from build123d import *

# Parameters (mm, degrees)
SKETCH2_W                      = 230
SKETCH2_H                      = 283.251
BOSS_EXTRUDE1_DEPTH            = 10
SKETCH3_W                      = 10
SKETCH3_H                      = 283.251
BOSS_EXTRUDE2_DEPTH            = 170
M6_CLEARANCE_HOLE1_D           = 7
CUT_EXTRUDE1_DEPTH             = 327.431895271
CUT_EXTRUDE1_DEPTH_BACK        = 327.431895271
SKETCH7_R                      = 3.81
SKETCH7_R_2                    = 1.89865
SKETCH8_W                      = 6.35
SKETCH8_H                      = 38.1
CUT_EXTRUDE2_DEPTH             = 36.025
CUT_EXTRUDE3_DEPTH             = 6.35
CUT_EXTRUDE4_REACH             = 331.125
SKETCH11_R                     = 3.81
F_6_CLEARANCE_HOLE1_D          = 3.7973
F_6_CLEARANCE_HOLE1_DEPTH      = 3.65
CIRPATTERN1_COUNT              = 2
ENL_V_MAT_EXTRU_1_REACH        = 249.554
ESQUISSE1_R                    = 3.175
CBORE_FOR_M5_SHCS1_D           = 5.5
CBORE_FOR_M5_SHCS1_CBORE_D     = 10
CBORE_FOR_M5_SHCS1_CBORE_DEPTH = 5
CUT_EXTRUDE5_DEPTH             = 248.553594703
CUT_EXTRUDE5_DEPTH_BACK        = 248.553594703
SKETCH15_W                     = 58.825
SKETCH15_H                     = 30.860637148
CUT_EXTRUDE7_DEPTH             = 248.553594703
CUT_EXTRUDE7_DEPTH_BACK        = 248.553594703
SKETCH20_W                     = 0.765
SKETCH20_H                     = 30.860637148
FILLET2_R                      = 4
FILLET3_R                      = 144
FILLET4_R                      = 4
CUT_EXTRUDE8_REACH             = 335.853
CUT_EXTRUDE9_REACH             = 335.853
FILLET5_R                      = 8
FILLET6_R                      = 8


with BuildPart() as part:
    # Sketch2 → Boss-Extrude1 (new body)
    with BuildSketch(Plane(origin=(0, 0, 0), x_dir=(1, 0, 0), z_dir=(0, 1, 0))):
        Rectangle(SKETCH2_W, SKETCH2_H)
    extrude(amount=BOSS_EXTRUDE1_DEPTH)

    # Sketch3 → Boss-Extrude2 (add)
    with BuildSketch(Plane(origin=(0, 0, 0), x_dir=(1, 0, 0), z_dir=(0, 1, 0))):
        with Locations((-120, 0)):
            Rectangle(SKETCH3_W, SKETCH3_H)
        with Locations((120, 0)):
            Rectangle(SKETCH3_W, SKETCH3_H)
    extrude(amount=BOSS_EXTRUDE2_DEPTH)

    # M6 Clearance Hole1 (through all)
    with Locations(Plane(origin=(0, 10, 0), x_dir=(1, 0, 0), z_dir=(0, 1, 0))):
        with Locations((-25, 25), (25, 25), (25, -25), (-25, -25)):
            Hole(M6_CLEARANCE_HOLE1_D / 2)

    # Sketch7 → Cut-Extrude1 (cut, two sides: drawn at the far end of the back side and taken through both)
    with BuildSketch(Plane.ZY.offset(-115).offset(-CUT_EXTRUDE1_DEPTH_BACK)):
        with Locations((0, 153.49)):
            Circle(SKETCH7_R)
        with Locations((0, 163.269)):
            Circle(SKETCH7_R_2)
        with Locations((6.914797213, 160.404797213)):
            Circle(SKETCH7_R_2)
        with Locations((9.779, 153.49)):
            Circle(SKETCH7_R_2)
        with Locations((6.914797213, 146.575202787)):
            Circle(SKETCH7_R_2)
        with Locations((0, 143.711)):
            Circle(SKETCH7_R_2)
        with Locations((-6.914797213, 146.575202787)):
            Circle(SKETCH7_R_2)
        with Locations((-9.779, 153.49)):
            Circle(SKETCH7_R_2)
        with Locations((-6.914797213, 160.404797213)):
            Circle(SKETCH7_R_2)
    extrude(amount=CUT_EXTRUDE1_DEPTH + CUT_EXTRUDE1_DEPTH_BACK, mode=Mode.SUBTRACT)

    # Sketch8 → Cut-Extrude2 (cut)
    with BuildSketch(Plane(origin=(0, 170, 0), x_dir=(1, 0, 0), z_dir=(0, 1, 0))):
        with Locations((121.825, 0)):
            Rectangle(SKETCH8_W, SKETCH8_H)
        with Locations((-121.825, 0)):
            Rectangle(SKETCH8_W, SKETCH8_H)
    extrude(amount=-CUT_EXTRUDE2_DEPTH, mode=Mode.SUBTRACT)

    # Sketch9 → Cut-Extrude3 (cut)
    with BuildSketch(Plane(origin=(125, 0, 0), x_dir=(0, 0, -1), z_dir=(1, 0, 0))):
        Polygon((100.764862852, 96.554), (100.764862852, 58.026), (62.744862852, 58.026), (62.744862852, 96.554), (62.744862852, 170), (100.764862852, 170), align=None)
    cut_extrude3 = extrude(amount=-CUT_EXTRUDE3_DEPTH, mode=Mode.SUBTRACT)

    # Sketch11 → Cut-Extrude4 (cut, up to next)
    with BuildSketch(Plane(origin=(118.65, 0, 0), x_dir=(0, 0, -1), z_dir=(1, 0, 0)), mode=Mode.PRIVATE) as cut_extrude4_sk1:
        with Locations((81.754862852, 77.29)):
            Circle(SKETCH11_R)
    cut_extrude4_tool1 = extrude(cut_extrude4_sk1.sketch, amount=-CUT_EXTRUDE4_REACH, mode=Mode.PRIVATE) & part.part
    cut_extrude4 = cut_extrude4_tool1.solids().sort_by_distance((118.65, 77.29, -81.754863))[0]
    add(cut_extrude4, mode=Mode.SUBTRACT)

    # #6 Clearance Hole1
    with Locations(Plane(origin=(118.65, 0, 0), x_dir=(0, 0, -1), z_dir=(1, 0, 0))):
        with Locations((81.754862852, 87.069), (71.975862852, 77.29), (91.533862852, 77.29), (81.754862852, 67.511)):
            f_6_clearance_hole1 = Hole(F_6_CLEARANCE_HOLE1_D / 2, depth=F_6_CLEARANCE_HOLE1_DEPTH)

    # CirPattern1: Cut-Extrude3, Cut-Extrude4, #6 Clearance Hole1 ×2 about axis
    cirpattern1_axis = Axis((0, 0, 0), (0, 1, 0))
    add([cut_extrude3.rotate(cirpattern1_axis, i * 360 / CIRPATTERN1_COUNT) for i in range(1, CIRPATTERN1_COUNT)], mode=Mode.SUBTRACT)
    add([cut_extrude4.rotate(cirpattern1_axis, i * 360 / CIRPATTERN1_COUNT) for i in range(1, CIRPATTERN1_COUNT)], mode=Mode.SUBTRACT)
    add([f_6_clearance_hole1.rotate(cirpattern1_axis, i * 360 / CIRPATTERN1_COUNT) for i in range(1, CIRPATTERN1_COUNT)], mode=Mode.SUBTRACT)

    # Esquisse1 → Enlèv. mat.-Extru.1 (cut, up to next)
    with BuildSketch(Plane(origin=(0, 10, 0), x_dir=(1, 0, 0), z_dir=(0, 1, 0)), mode=Mode.PRIVATE) as enl_v_mat_extru_1_sk1:
        with Locations(Location((53, 110.739314032, 0), (0, 0, 270))):
            Circle(ESQUISSE1_R)
    enl_v_mat_extru_1_tool1 = extrude(enl_v_mat_extru_1_sk1.sketch, amount=-ENL_V_MAT_EXTRU_1_REACH, mode=Mode.PRIVATE) & part.part
    # Esquisse1 → Enlèv. mat.-Extru.1 (cut, up to next)
    with BuildSketch(Plane(origin=(0, 10, 0), x_dir=(1, 0, 0), z_dir=(0, 1, 0)), mode=Mode.PRIVATE) as enl_v_mat_extru_1_sk2:
        with Locations(Location((53, 10.203163452, 0), (0, 0, 270))):
            Circle(ESQUISSE1_R)
    enl_v_mat_extru_1_tool2 = extrude(enl_v_mat_extru_1_sk2.sketch, amount=-ENL_V_MAT_EXTRU_1_REACH, mode=Mode.PRIVATE) & part.part
    add(enl_v_mat_extru_1_tool1.solids().sort_by_distance((53, 10, -110.739314))[0], mode=Mode.SUBTRACT)
    add(enl_v_mat_extru_1_tool2.solids().sort_by_distance((53, 10, -10.203163))[0], mode=Mode.SUBTRACT)

    # CBORE for M5 SHCS1 (through all)
    with Locations(Plane(origin=(0, 0, 0), x_dir=(-1, 0, 0), z_dir=(0, -1, 0))):
        with Locations((53, -52.770411672), (53, -153.306562253)):
            CounterBoreHole(CBORE_FOR_M5_SHCS1_D / 2, CBORE_FOR_M5_SHCS1_CBORE_D / 2, CBORE_FOR_M5_SHCS1_CBORE_DEPTH)

    # Sketch15 → Cut-Extrude5 (cut, two sides: drawn at the far end of the back side and taken through both)
    with BuildSketch(Plane(origin=(0, 10, 0), x_dir=(1, 0, 0), z_dir=(0, 1, 0)).offset(-CUT_EXTRUDE5_DEPTH_BACK)):
        with BuildLine():
            Line((125, 141.6255), (-125, 141.6255))
            Line((-125, 141.6255), (-125, 29.05))
            Line((-125, 29.05), (-82.580571034, 29.05))
            ThreePointArc((-82.580571034, 29.05), (-32.48081845, 81.292371383), (39.825, 77.957825696))
            Line((39.825, 77.957825696), (39.825, 123.914314032))
            Line((39.825, 123.914314032), (66.175, 123.914314032))
            Line((66.175, 123.914314032), (66.175, 110.764862852))
            Line((66.175, 110.764862852), (125, 110.764862852))
            Line((125, 110.764862852), (125, 141.6255))
        make_face()
        with BuildLine():
            Line((125, -141.6255), (125, -29.05))
            Line((125, -29.05), (82.580571034, -29.05))
            ThreePointArc((82.580571034, -29.05), (32.48081845, -81.292371383), (-39.825, -77.957825696))
            Line((-39.825, -77.957825696), (-39.825, -141.6255))
            Line((-39.825, -141.6255), (125, -141.6255))
        make_face()
        with Locations((-95.5875, -126.195181426)):
            Rectangle(SKETCH15_W, SKETCH15_H)
    extrude(amount=CUT_EXTRUDE5_DEPTH + CUT_EXTRUDE5_DEPTH_BACK, mode=Mode.SUBTRACT)

    # Sketch20 → Cut-Extrude7 (cut, two sides: drawn at the far end of the back side and taken through both)
    with BuildSketch(Plane(origin=(0, 10, 0), x_dir=(1, 0, 0), z_dir=(0, 1, 0)).offset(-CUT_EXTRUDE7_DEPTH_BACK)):
        with Locations((-65.7925, -126.195181426)):
            Rectangle(SKETCH20_W, SKETCH20_H)
        with BuildLine():
            Line((-39.825, -141.6255), (-39.825, -107.748743461))
            ThreePointArc((-39.825, -107.748743461), (-41.410278355, -109.222344653), (-41.995854347, -111.306021378))
            Line((-41.995854347, -111.306021378), (-41.995854347, -141.6255))
            Line((-41.995854347, -141.6255), (-39.825, -141.6255))
        make_face()
        with BuildLine():
            Line((39.825, 123.914314032), (66.175, 123.914314032))
            Line((66.175, 123.914314032), (66.175, 110.764862852))
            Line((66.175, 110.764862852), (65.41, 110.764862852))
            Line((65.41, 110.764862852), (65.41, 116.58385488))
            ThreePointArc((65.41, 116.58385488), (64.238427125, 119.412282005), (61.41, 120.58385488))
            Line((61.41, 120.58385488), (46, 120.58385488))
            ThreePointArc((46, 120.58385488), (43.171572875, 119.412282005), (42, 116.58385488))
            Line((42, 116.58385488), (42, 104.58385488))
            ThreePointArc((42, 104.58385488), (41.413209633, 102.498189519), (39.825, 101.024448329))
            Line((39.825, 101.024448329), (39.825, 123.914314032))
        make_face()
    extrude(amount=CUT_EXTRUDE7_DEPTH + CUT_EXTRUDE7_DEPTH_BACK, mode=Mode.SUBTRACT)

    # Fillet2
    fillet2_edges = [part.edges().sort_by_distance(p)[0] for p in [
        (-65.41, 5, 141.6255),
        (-41.995854347, 5, 141.6255),
    ]]
    fillet(fillet2_edges, radius=FILLET2_R)

    # Fillet3
    # the kernel refuses this fillet: 144 mm, written as the material it adds along each edge
    with BuildSketch(Plane(origin=(39.825, 0, -77.957825696), x_dir=(-0.9828868635298122, 0, -0.18421024265911018), z_dir=(0, 1, 0))) as fillet3_piece_1:
        with BuildLine():
            CenterArc((90.33197894, -138.109046644), FILLET3_R, 106.445268475, 20.267064332)
            Line((4.249108153, -22.671880372), (2.527450737, -20.363137046))
            ThreePointArc((2.527450737, -20.363137046), (-0.706160091, -11.866465685), (-2.830714167, -0.530525499))
            Line((-2.830714167, -0.530525499), (0.815326005, 2.762180933))
            ThreePointArc((0.815326005, 2.762180933), (24.782839351, -0.701255836), (48.750352698, 2.762180933))
            Line((48.750352698, 2.762180933), (49.565678703, 0))
        make_face()
    extrude(amount=10)
    with BuildSketch(Plane(origin=(-39.825, 10, 77.957825696), x_dir=(0, 0, 1), z_dir=(0, -1, 0))) as fillet3_piece_2:
        with BuildLine():
            CenterArc((150.266135455, -78.877892483), FILLET3_R, 146.786309889, 23.503480659)
            Line((8.329161454, -54.590129896), (5.490421974, -54.104374645))
            ThreePointArc((5.490421974, -54.104374645), (5.734767963, -27.055491549), (-2.564719952, -1.310195239))
            Line((-2.564719952, -1.310195239), (0, 2.88))
            ThreePointArc((0, 2.88), (14.895458882, 2.88), (27.381413411, 1.57755785))
            Line((27.381413411, 1.57755785), (29.790917765, 0))
        make_face()
    extrude(amount=10)

    # Fillet4
    fillet4_edges = [part.edges().sort_by_distance(p)[0] for p in [
        (-82.580571034, 5, -29.05),
        (82.580571034, 5, 29.05),
        (-65.41, 5, 110.764862852),
        (65.41, 5, -110.764862852),
    ]]
    fillet(fillet4_edges, radius=FILLET4_R)

    # Sketch22 → Cut-Extrude8 (cut, up to next)
    with BuildSketch(Plane.ZY.offset(125), mode=Mode.PRIVATE) as cut_extrude8_sk1:
        Polygon((40.857431426, 170), (110.764862852, 104.051), (110.764862852, 170), align=None)
    cut_extrude8_tool1 = extrude(cut_extrude8_sk1.sketch, amount=-CUT_EXTRUDE8_REACH, mode=Mode.PRIVATE) & part.part
    add(cut_extrude8_tool1.solids().sort_by_distance((-125, 148.017, 87.462386))[0], mode=Mode.SUBTRACT)

    # Sketch23 → Cut-Extrude9 (cut, up to next)
    with BuildSketch(Plane(origin=(125, 0, 0), x_dir=(0, 0, -1), z_dir=(1, 0, 0)), mode=Mode.PRIVATE) as cut_extrude9_sk1:
        Polygon((29.05, 170), (110.764862852, 104.051), (110.764862852, 170), align=None)
    cut_extrude9_tool1 = extrude(cut_extrude9_sk1.sketch, amount=-CUT_EXTRUDE9_REACH, mode=Mode.PRIVATE) & part.part
    add(cut_extrude9_tool1.solids().sort_by_distance((125, 148.017, -83.526575))[0], mode=Mode.SUBTRACT)

    # Fillet5
    fillet5_edges = [part.edges().sort_by_distance(p)[0] for p in [
        (-120, 170, -29.05),
        (120, 170, 29.05),
        (-120, 170, 40.857431426),
        (-120, 104.051, 110.764862852),
        (120, 170, -29.05),
        (120, 104.051, -110.764862852),
    ]]
    fillet(fillet5_edges, radius=FILLET5_R)

    # Fillet6
    fillet6_edges = [part.edges().sort_by_distance(p)[0] for p in [
        (-121.825, 149.351920308, 62.744862852),
    ]]
    fillet(fillet6_edges, radius=FILLET6_R)


solid = part.part
Work out the finished part from the listing and answer in its coordinate system (mm). A direction names the side the tool comes from. Coordinates: 2 decimals unless noted, no trailing zeros. Write each loop counter-clockwise with the first axis right and the second up, starting at its lowest first coordinate (ties: lowest second). Pieces come first, ordered by that corner, then holes. Notation, with made-up numbers: M 73.25,19 L 78.25,19 A11 cw 78.25,31 Z; hole C 62.5,42 d8. An arc over 180 degrees is marked long. Answer as CSV lines item,"result". Start each with the question number.
Item 1: Section B-B on z = 25 is taken. Write down the section's boundary in (x, y), and give its area (3 significant figures).
Item 2: Consider L1, parallel to Y at x = 117, z = 0; L2, parallel to X at y = 127, z = -1; L3, parallel to Y at x = 57, z = -4. Determine where each line is inside the solid, lowest interval first.
Item 3: Section A-A on y = 43 is taken. Write down the section's boundary in (x, z), and give its area (3 significant figures).
Item 4: Flat-ended cylindrical pins translate along their axes: P1, Ø3.5, axis at y = 163.269, z = 0, coming from the -X side; P2, Ø6, axis at y = 160.4, z = 6.91, coming from the +X side; P3, Ø1.9, axis at x = -121, y = 95, coming from the -Z side; P4, Ø3, axis at x = 120.5, y = 92, coming from the +Z side. Find the tip coordinate at first contact, or state that the pin passes through.
Item 5: Determine the mould class of faces 6 (the face through (42, 5, -111)), 7 (the face through (-117.848, 137.549, 75.256)), 8 (the face through (122, 85, -100.765)), 9 (the face through (122, 152, 19.05)) for opening direction Z: released by +Z, released by -Z, zero draft, split by the parting line, or undercut.
Item 6: A tool of negligible diameter and unlimited length cuts with its end or side. For faces 1 (the face through (-41.996, 5, 124)), 2 (the face through (-122, 85, 100.765)), 3 (the face through (118.65, 148, 0)), 4 (the face through (120.07, 167.594, 26.769)), 5 (the face through (115, 89, -40)), from which of +Z, -Z, +X, -X, +Y, -Y can it reach the whole face along a straight path? Write none if from no direction.
Checks:
1,outline,"M -125,0 L -28.5,0 L -28.5,10 L -115,10 L -115,170 L -125,170 Z; M -21.5,0 L 21.5,0 L 21.5,10 L -21.5,10 Z; M 28.5,0 L 125,0 L 125,168.96 L 115,168.96 L 115,10 L 28.5,10 Z"
1,area,"5,550 mm²"
2,L1,"y = 0 to 141.81, 145.61 to 149.68, 157.3 to 161.37, 165.17 to 170"
2,L2,"x = -125 to -115, 115 to 125"
2,L3,"y = 0 to 10"
3,outline,"M -125,-29.05 L -115,-29.05 L -115,110.76 L -125,110.76 Z; M 115,-110.76 L 125,-110.76 L 125,29.05 L 115,29.05 Z"
3,area,"2,800 mm²"
4,P1,"passes through"
4,P2,"stops at x = 118.65"
4,P3,"stops at z = -29.05"
4,P4,"stops at z = 29.05"
5,face 6,"zero draft"
5,face 7,"released by +Z"
5,face 8,"undercut"
5,face 9,"undercut"
6,face 1,"+Z, +X, +Y, -Y"
6,face 2,"-X, +Y"
6,face 3,"+X, +Y"
6,face 4,"+Z, +X, +Y"
6,face 5,"+Z, -Z, +Y"
